Design review of the part built by this model. Coordinates are the model's own, in mm. A direction names the side the tool comes from. Give positions to 0.01 mm unless a question says otherwise; leave off trailing zeros. Loops run counter-clockwise (first coordinate to the right, second up) from the corner with the lowest first, then second, coordinate; pieces in that order, holes last. Notation, with made-up numbers: (62.5, 23.5) -> (120.5, 23.5) arc R35 ccw to (120.5, 55.5) -> close; hole circle Ø8 at (24, 69). An arc over 180 degrees is marked (long way). Use a Markdown table: item, result. Add a question column.
1. Add section D-D (z = -10). State the section outline as (x, y) points, and give its area (3 significant figures).
2. Add section A-A (z = -15.5). State the section outline as (x, y) points, and give its area (3 significant figures).
3. For pin 1 Ø2.5 at (x, y) = (0, -10) entering from +Z; pin 2 Ø2 at (x, y) = (0, -20) entering from +Z; pin 3 Ø3 at (x, z) = (0.5, 17.5) entering from -Y; pin 4 Ø2.5 at (x, y) = (0, 16) entering from +Z, all flat-tipped, find the tip position at first contact; note any pin that passes through.
4. Draft analysis for pull direction X (two halves, no side actions). For faces 4 (the flat face through (2.5, 4.8, -16.2)), 5 (the flat face through (2.3, -22, -9.9)), 6 (the cylindrical face through (0, 8, -18)), state which applies: pulls with the +X half, pulls with the -X half, needs draft (parallel to the pull), parting line crosses it, or undercut.
5. Add section C-C (y = -10). State the section outline as (x, z) points.
6. To check wall thickness, follow line 1 (Z direction, x = 0, y = 20.6); line 2 (Y direction, x = 0, z = -17.5); line 3 (X direction, y = -10, z = -17.5). State the ranges of each line that lie inside material, in increasing order.
7. For faces 1 (the cylindrical face through (0, 18, 18)), 2 (the flat face through (1, -18, -8)), 3 (the flat face through (0, -20, 0)), list the 3-axis set-ups (+Z, -Z, +X, -X, +Y, -Y) from which the entire face can be reached by the end or side of a thin tool; tool diameter is ignored.
8. Add section B-B (y = 16). State the section outline as (x, z) points.
```python
from build123d import *

# Parameters (mm, degrees)
F1_DEPTH = 2.5
F2_R     = 2
F3_DEPTH = 5
F4_R     = 2
F5_DEPTH = 5
F6_R     = 2
F7_DEPTH = 25
F8_R     = 2
F9_DEPTH = 5


with BuildPart() as f1:
    # F0 (on Right) → F1 (new body, symmetric)
    with BuildSketch(Plane.YZ):
        Polygon((-22, -20), (22, -20), (22, 20), (12, 20), (12, 16), (18, 16), (18, -16), (-18, -16), (-18, 0), (-22, 0), align=None)
    extrude(amount=F1_DEPTH, both=True)

    # F2 (on face) → F3 (cut)
    with BuildSketch(Plane.XY.offset(20)):
        with Locations((0, 16)):
            Circle(F2_R)
    extrude(amount=-F3_DEPTH, mode=Mode.SUBTRACT)

    # F4 (on face) → F5 (cut)
    with BuildSketch(Plane(origin=(0, 0, -20), x_dir=(1, 0, 0), z_dir=(0, 0, -1))):
        with Locations((0, 10)):
            Circle(F4_R)
        with Locations((0, -10)):
            Circle(F4_R)
    extrude(amount=-F5_DEPTH, mode=Mode.SUBTRACT)

    # F6 (on face) → F7 (cut)
    with BuildSketch(Plane.XZ.offset(22)):
        with Locations((0, -10)):
            Circle(F6_R)
    extrude(amount=-F7_DEPTH, mode=Mode.SUBTRACT)

    # F8 (on face) → F9 (cut)
    with BuildSketch(Plane(origin=(0, 22, 0), x_dir=(-1, 0, 0), z_dir=(0, 1, 0))):
        with Locations((0, -10)):
            Circle(F8_R)
        with Locations((0, 10)):
            Circle(F8_R)
    extrude(amount=-F9_DEPTH, mode=Mode.SUBTRACT)


solid = f1.part
```
Taken from the geometry:
| question | item | result |
|---|---|---|
| 1 | outline | (-2.5, -22) -> (-2, -22) -> (-2, -18) -> (-2.5, -18) -> close; (-2.5, 18) -> (-2, 18) -> (-2, 22) -> (-2.5, 22) -> close; (2, -22) -> (2.5, -22) -> (2.5, -18) -> (2, -18) -> close; (2, 18) -> (2.5, 18) -> (2.5, 22) -> (2, 22) -> close |
| 1 | area | 8.00 mm^2 |
| 2 | outline | (-2.5, -22) -> (2.5, -22) -> (2.5, -18) -> (-2.5, -18) -> close; (-2.5, 18) -> (2.5, 18) -> (2.5, 22) -> (-2.5, 22) -> close |
| 2 | area | 40.0 mm^2 |
| 3 | pin 1 | passes through |
| 3 | pin 2 | stops at z = 0 |
| 3 | pin 3 | stops at y = 12 |
| 3 | pin 4 | stops at z = -16 |
| 4 | face 4 | pulls with the +X half |
| 4 | face 5 | needs draft |
| 4 | face 6 | undercut |
| 5 | outline | (-2.5, -20) -> (-2, -20) -> (-2, -16) -> (-2.5, -16) -> close; (2, -20) -> (2.5, -20) -> (2.5, -16) -> (2, -16) -> close |
| 6 | line 1 | z = -20 to -12, -8 to 8, 12 to 20 |
| 6 | line 2 | y = -22 to -12, -8 to 8, 12 to 22 |
| 6 | line 3 | x = -2.5 to -2, 2 to 2.5 |
| 7 | face 1 | +Z |
| 7 | face 2 | +Z, +X, -X |
| 7 | face 3 | +Z, +X, -X, -Y |
| 8 | outline | (-2.5, -20) -> (2.5, -20) -> (2.5, -16) -> (-2.5, -16) -> close; (-2.5, 16) -> (-2, 16) -> (-2, 20) -> (-2.5, 20) -> close; (2, 16) -> (2.5, 16) -> (2.5, 20) -> (2, 20) -> close |
